from build123d import *

# Parameters (mm, degrees)
F0_R     = 7.5
F0_R_2   = 2.5
F1_DEPTH = 4
F2_DEPTH = 10
F3_R     = 0.5


with BuildPart() as f1:
    # F0 (on Top) → F1 (new body)
    with BuildSketch(Plane.XY):
        Circle(F0_R)
        Circle(F0_R_2, mode=Mode.SUBTRACT)
        Circle(F0_R_2)
    extrude(amount=F1_DEPTH)

    # F0 (on Top) → F2 (join)
    with BuildSketch(Plane.XY):
        Circle(F0_R_2)
    extrude(amount=F2_DEPTH)

    # F3
    f3_edges = [f1.edges().sort_by_distance(p)[0] for p in [
        (-7.5, 0, 4),
        (-7.5, 0, 0),
        (-2.5, 0, 10),
        (-2.5, 0, 4),
    ]]
    fillet(f3_edges, radius=F3_R)


solid = f1.part
Check sheet for the modelled part. Datum: model origin and axes. Units: mm. A direction names the side the tool comes from. Round coordinates to 2 decimals unless told otherwise and drop trailing zeros. Write each loop counter-clockwise with the first axis right and the second up, starting at its lowest first coordinate (ties: lowest second). Pieces come first, ordered by that corner, then holes. Notation, with made-up numbers: (7, 12.5) -> (64, 12.5) arc R24 ccw to (64, 27.5) -> close; hole circle Ø5 at (-40, 73). An arc over 180 degrees is marked (long way). Answer as CSV lines item,"result". Start each with the question number.
1) Section check D-D on z = 3. Enter the section's corners in (x, y), and give its area (3 significant figures).
2) Go/stop test with flat-tipped pins: P1, Ø7, axis at x = 0, y = -3, coming from the +Z side; P2, Ø4, axis at x = -6, y = 3.5, coming from the +Z side; P3, Ø1.5, axis at y = -5, z = 8.5, coming from the +X side; P4, Ø3, axis at y = 0.5, z = 9, coming from the -X side. Record where each tip stops, or that it passes through.
3) Material ranges on line 1 (X direction, y = 1.5, z = 5.5); line 2 (Z direction, x = 1.5, y = 5.75); line 3 (X direction, y = -1, z = 4.5), recorded low to high. Write a range as from..to.
4) Section check C-C on z = 5. Enter the section's corners in (x, y), and give its area (3 significant figures).
5) Tool access check on faces 1 (the flat face through (1, -3, 4)), 2 (the cylindrical face through (-7.493, 0.33, 1.979)). Record the directions out of +Z, -Z, +X, -X, +Y, -Y that give a thin tool (end or side, any length) a straight path to the whole face; none if there is none.
6) Section check A-A on y = 0. Enter the section's corners in (x, z), and give its area (3 significant figures).
Found:
1,outline,"circle Ø15 at (0, 0)"
1,area,"177 mm^2"
2,P1,"stops at z = 10"
2,P2,"stops at z = 4"
2,P3,"passes through"
2,P4,"stops at x = -2.5"
3,line 1,"x = -2..2"
3,line 2,"z = 0..4"
3,line 3,"x = -2.29..2.29"
4,outline,"circle Ø5 at (0, 0)"
4,area,"19.6 mm^2"
5,face 1,"+Z"
5,face 2,"+Z, -Z"
6,outline,"(-7.5, 0.5) arc R0.5 ccw to (-7, 0) -> (7, 0) arc R0.5 ccw to (7.5, 0.5) -> (7.5, 3.5) arc R0.5 ccw to (7, 4) -> (3, 4) arc R0.5 cw to (2.5, 4.5) -> (2.5, 9.5) arc R0.5 ccw to (2, 10) -> (-2, 10) arc R0.5 ccw to (-2.5, 9.5) -> (-2.5, 4.5) arc R0.5 cw to (-3, 4) -> (-7, 4) arc R0.5 ccw to (-7.5, 3.5) -> close"
6,area,"89.8 mm^2"
